Part model, mm, in its own coordinate system. A direction names the side the tool comes from. Round coordinates to 2 decimals unless told otherwise and drop trailing zeros. Loops run counter-clockwise (first coordinate to the right, second up) from the corner with the lowest first, then second, coordinate; pieces in that order, holes last. Notation, with made-up numbers: (16.5, 0.5) - (58.5, 0.5) arc R8 ccw to (58.5, 7.5) - close; hole circle Ø4 at (62, 15.5). An arc over 180 degrees is marked (long way). Put each result on its own line as item: value.
from build123d import *

# Parameters (mm, degrees)
BOSS_EXTRU_1_DEPTH      = 1.4
BOSS_EXTRU_2_START      = -7
ESQUISSE2_R             = 5.4
ESQUISSE2_R_2           = 4.1
BOSS_EXTRU_2_DEPTH      = 7
ENL_V_MAT_EXTRU_1_DEPTH = 7


with BuildPart() as part:
    # Esquisse1 → Boss.-Extru.1 (new body)
    with BuildSketch(Plane.XY):
        with BuildLine():
            Line((4.1, 0), (4.1, 12.757350822))
            ThreePointArc((4.1, 12.757350822), (0, -13.4), (-4.1, 12.757350822))
            Line((-4.1, 12.757350822), (-4.1, 0))
            ThreePointArc((-4.1, 0), (0, -4.1), (4.1, 0))
        make_face()
    extrude(amount=BOSS_EXTRU_1_DEPTH)

    # Esquisse2 → Boss.-Extru.2 (add)
    with BuildSketch(Plane.XY.offset(1.4).offset(BOSS_EXTRU_2_START)):
        Circle(ESQUISSE2_R)
        Circle(ESQUISSE2_R_2, mode=Mode.SUBTRACT)
    extrude(amount=BOSS_EXTRU_2_DEPTH)

    # Esquisse3 → Enlèv. mat.-Extru.1 (cut)
    with BuildSketch(Plane(origin=(0, 0, 0), x_dir=(1, 0, 0), z_dir=(0, 1, 0))):
        with BuildLine():
            Line((-4.1, -1.4), (-4.1, 0))
            ThreePointArc((-4.1, 0), (0, 4.1), (4.1, 0))
            Line((4.1, 0), (4.1, -1.4))
            Line((4.1, -1.4), (-4.1, -1.4))
        make_face()
    extrude(amount=ENL_V_MAT_EXTRU_1_DEPTH, mode=Mode.SUBTRACT)


solid = part.part
1. Two-plate mould, pull along Y, no slides. Class faces 4 (the cylindrical face through (0.53, -13.39, 0.69)), 5 (the cylindrical face through (-0.9, -4, -2.9)), 6 (the flat face through (-3.2, -3, 1.4)): pulls with the +Y half, pulls with the -Y half, needs draft (parallel to the pull), parting line crosses it, or undercut.
A:
face 4: parting line crosses it
face 5: undercut
face 6: needs draft
2. Pin check, flat tips, straight feed: P1, Ø1, axis at x = 5.5, y = -2, coming from the -Z side; P2, Ø1, axis at x = -4.5, z = -4, coming from the -Y side; P3, Ø1.1, axis at y = 7, z = 0.5, coming from the +X side; P4, Ø1.1, axis at y = 8.5, z = 1, coming from the -X side. Stop position of each tip, or through.
A:
P1: stops at z = -5.6
P2: stops at y = -3.63
P3: stops at x = 11.75
P4: stops at x = -10.79
3. Band-saw the part on B-B (y = 2.5). List the corners of the cut face in (x, z).
A:
outline: (-13.16, 0) - (-4.79, 0) - (-4.79, -5.6) - (-3.25, -5.6) - (-3.25, -2.5) arc R4.1 cw to (-4.1, 0) - (-4.1, 1.4) - (-13.16, 1.4) - close; (3.25, -5.6) - (4.79, -5.6) - (4.79, 0) - (13.16, 0) - (13.16, 1.4) - (4.1, 1.4) - (4.1, 0) arc R4.1 cw to (3.25, -2.5) - close
4. Band-saw the part on D-D (x = -4.5). List the corners of the cut face in (y, z).
A:
outline: (-12.62, 0) - (-2.98, 0) - (-2.98, -5.6) - (2.98, -5.6) - (2.98, 0) - (12.62, 0) - (12.62, 1.4) - (-12.62, 1.4) - close
5. Band-saw the part on C-C (x = 3.25). List the corners of the cut face in (y, z), plus the area to 3 significant figures.
A:
outline: (-13, 0) - (-4.31, 0) - (-4.31, -5.6) - (-2.5, -5.6) - (-2.5, 1.4) - (-13, 1.4) - close; (2.5, -5.6) - (4.31, -5.6) - (4.31, -2.5) - (2.5, -2.5) - close
area: 30.5 mm²
6. Tool access for faces 1 (the flat face through (4.1, 6, 1)), 2 (the cylindrical face through (-1.17, -5.27, -2.84)), 3 (the flat face through (4, 2, -5.6)): list every direction of +Z, -Z, +X, -X, +Y, -Y with a clear straight run to the whole face (end or side of a thin tool).
A:
face 1: +Z, +Y
face 2: -Z
face 3: -Z, +X, -X, +Y, -Y
7. Band-saw the part on A-A (x = 0). List the corners of the cut face in (y, z).
A:
outline: (-13.4, 0) - (-5.4, 0) - (-5.4, -5.6) - (-4.1, -5.6) - (-4.1, 1.4) - (-13.4, 1.4) - close; (4.1, -5.6) - (5.4, -5.6) - (5.4, -4.1) - (4.1, -4.1) - close
8. Probe line 1 along X through (y, z) = (0, -1.75); line 2 along X through (y, z) = (0, 0.25); line 3 along Z through (x, y) = (9.5, -2.25). List the from-to ranges inside material, lowest first. Write a range as [from, to].
A:
line 1: x = [-5.4, -4.1], [4.1, 5.4]
line 2: x = [-13.4, -4.1], [4.1, 13.4]
line 3: z = [0, 1.4]
